Input: part model. Units: mm. Frame: model coordinates. A direction names the side the tool comes from. Give positions to 0.01 mm unless a question says otherwise; leave off trailing zeros. Order: outer loops, then holes, each group sorted by start corner. A loop starts at its lowest first (then second) coordinate and runs counter-clockwise, first axis right, second up. Notation, with made-up numbers: M 8,-2 L 48,-2 A33 ccw 48,32 Z; hole C 28.5,10.25 d11. An arc over 180 degrees is marked long. Use a Markdown table: item, result.
from build123d import *

# Parameters (mm, degrees)
EXTRUDE_3_DEPTH     = 80
SHELL_14_T          = -3
CUT_EXTRUDE_1_REACH = 170.526
SKETCH_9_R          = 2.6
EXTRUDE_7_REACH     = 169.123
CUT_EXTRUDE_2_REACH = 185.868
SKETCH_24_R         = 5.05


with BuildPart() as part:
    # 草图5 → 凸台-拉伸3 (new body)
    with BuildSketch(Plane.XY):
        Polygon((0, 49), (0, 0), (80, -42.359693068), (140, -42.359693068), align=None)
    extrude(amount=EXTRUDE_3_DEPTH)

    # 抽壳14
    shell_14_openings = [part.faces().sort_by_distance(p)[0] for p in [
        (70, 3.320153466, 40),
    ]]
    offset(amount=SHELL_14_T, openings=shell_14_openings, kind=Kind.INTERSECTION)

    # 草图9 → 切除-拉伸1 (cut, up to next)
    with BuildSketch(Plane.ZY, mode=Mode.PRIVATE) as cut_extrude_1_sk1:
        with Locations(Location((70, 9.5, 0), (0, 0, 270))):
            Circle(SKETCH_9_R)
    cut_extrude_1_tool1 = extrude(cut_extrude_1_sk1.sketch, amount=-CUT_EXTRUDE_1_REACH, mode=Mode.PRIVATE) & part.part
    # 草图9 → 切除-拉伸1 (cut, up to next)
    with BuildSketch(Plane.ZY, mode=Mode.PRIVATE) as cut_extrude_1_sk2:
        with Locations(Location((70, 39.5, 0), (0, 0, 270))):
            Circle(SKETCH_9_R)
    cut_extrude_1_tool2 = extrude(cut_extrude_1_sk2.sketch, amount=-CUT_EXTRUDE_1_REACH, mode=Mode.PRIVATE) & part.part
    # 草图9 → 切除-拉伸1 (cut, up to next)
    with BuildSketch(Plane.ZY, mode=Mode.PRIVATE) as cut_extrude_1_sk3:
        with Locations(Location((10, 9.5, 0), (0, 0, 270))):
            Circle(SKETCH_9_R)
    cut_extrude_1_tool3 = extrude(cut_extrude_1_sk3.sketch, amount=-CUT_EXTRUDE_1_REACH, mode=Mode.PRIVATE) & part.part
    # 草图9 → 切除-拉伸1 (cut, up to next)
    with BuildSketch(Plane.ZY, mode=Mode.PRIVATE) as cut_extrude_1_sk4:
        with Locations(Location((10, 39.5, 0), (0, 0, 270))):
            Circle(SKETCH_9_R)
    cut_extrude_1_tool4 = extrude(cut_extrude_1_sk4.sketch, amount=-CUT_EXTRUDE_1_REACH, mode=Mode.PRIVATE) & part.part
    add(cut_extrude_1_tool1.solids().sort_by_distance((0, 9.5, 70))[0], mode=Mode.SUBTRACT)
    add(cut_extrude_1_tool2.solids().sort_by_distance((0, 39.5, 70))[0], mode=Mode.SUBTRACT)
    add(cut_extrude_1_tool3.solids().sort_by_distance((0, 9.5, 10))[0], mode=Mode.SUBTRACT)
    add(cut_extrude_1_tool4.solids().sort_by_distance((0, 39.5, 10))[0], mode=Mode.SUBTRACT)

    # 草图23 → 凸台-拉伸7 (add, up to next)
    with BuildSketch(Plane.XY.offset(3), mode=Mode.PRIVATE) as extrude_7_sk1:
        Polygon((80.745233001, -39.359693068), (80.745233001, -3.691855026), (3, 1.806109525), align=None)
    extrude_7_tool1 = extrude(extrude_7_sk1.sketch, amount=EXTRUDE_7_REACH, mode=Mode.PRIVATE) - part.part
    add(extrude_7_tool1.solids().sort_by_distance((54.830155, -13.74848, 3))[0])

    # 草图24 → 切除-拉伸2 (cut, up to next)
    with BuildSketch(Plane(origin=(0, -39.359693068, 0), x_dir=(1, 0, 0), z_dir=(0, 1, 0)), mode=Mode.PRIVATE) as cut_extrude_2_sk1:
        with Locations(Location((115.745233001, -40, 0), (0, 0, 270))):
            Circle(SKETCH_24_R)
    cut_extrude_2_tool1 = extrude(cut_extrude_2_sk1.sketch, amount=-CUT_EXTRUDE_2_REACH, mode=Mode.PRIVATE) & part.part
    add(cut_extrude_2_tool1.solids().sort_by_distance((115.745233, -39.359693, 40))[0], mode=Mode.SUBTRACT)


solid = part.part
1) Reachability of faces 4 (the face through (42.42, -0.98, 39.48)), 5 (the face through (110, -42.36, 39)) from +Z, -Z, +X, -X, +Y, -Y: full face, straight path, thin tool, end or side. Return the list, or none.
Response values:
| item | result |
|---|---|
| face 4 | +X, +Y |
| face 5 | +Z, -Z, +X, -X, -Y |
2) Cut plane B-B on y = 40.5. Return loops of the section in (x, z).
Response values:
| item | result |
|---|---|
| outline | M 0,0 L 13.03,0 L 13.03,3 L 3,3 L 3,7.6 L 0,7.6 Z; M 0,12.4 L 3,12.4 L 3,67.6 L 0,67.6 Z; M 0,72.4 L 3,72.4 L 3,77 L 13.03,77 L 13.03,80 L 0,80 Z |
3) Mould query, pull axis Z, two halves, no side actions, for faces 1 (the face through (75.512, -0.277, 78.332)), 2 (the face through (1.479, 41.563, 8.418)), 3 (the face through (54, -10, 80)). Classes: released by +Z, released by -Z, zero draft, split by the parting line, or undercut.
Response values:
| item | result |
|---|---|
| face 1 | zero draft |
| face 2 | undercut |
| face 3 | released by +Z |
4) Cut plane C-C on z = 40. Return loops of the section in (x, y), and give its area (3 significant figures).
Response values:
| item | result |
|---|---|
| outline | M 0,0 L 80,-42.36 L 110.7,-42.36 L 110.7,-39.36 L 80.75,-39.36 L 80.75,-3.69 L 3,1.81 L 3,47.04 L 0,49 Z; M 120.8,-42.36 L 140,-42.36 L 135.4,-39.36 L 120.8,-39.36 Z |
| area | 1,940 mm² |
5) Cut plane A-A on z = 70. Return loops of the section in (x, y).
Response values:
| item | result |
|---|---|
| outline | M 0,0 L 80,-42.36 L 140,-42.36 L 135.4,-39.36 L 80.75,-39.36 L 80.75,-3.69 L 3,1.81 L 3,6.9 L 0,6.9 Z; M 0,12.1 L 3,12.1 L 3,36.9 L 0,36.9 Z; M 0,42.1 L 3,42.1 L 3,47.04 L 0,49 Z |
6) Material intervals for line 1 (Z direction, x = 1.25, y = 9.5); line 2 (Z direction, x = 58.5, y = 5.5); line 3 (Y direction, x = 96, z = 40), sorted ascending. Write a range as from..to.
Response values:
| item | result |
|---|---|
| line 1 | z = 0..7.4, 12.6..67.4, 72.6..80 |
| line 2 | z = 0..3, 77..80 |
| line 3 | y = -42.36..-39.36 |
7) First-contact query: pin 1 Ø7 at (y, z) = (9.5, 70) entering from +X; pin 2 Ø5 at (x, z) = (90.5, 44.5) entering from +Y; pin 3 Ø5 at (x, y) = (77.5, -2) entering from -Z; pin 4 Ø4.5 at (y, z) = (39.5, 70) entering from -X. Flat tips, straight axial feed; report the tip coordinate or a pass-through.
Response values:
| item | result |
|---|---|
| pin 1 | stops at x = 3 |
| pin 2 | stops at y = -39.36 |
| pin 3 | stops at z = 0 |
| pin 4 | passes through |
8) Cut plane D-D on x = 42. Return loops of the section in (y, z).
Response values:
| item | result |
|---|---|
| outline | M -22.24,0 L 21.59,0 L 21.59,3 L -0.95,3 L -0.95,77 L 21.59,77 L 21.59,80 L -22.24,80 Z |
